```python
from build123d import *

# Parameters (mm, degrees)
F0_R     = 2.0193
F0_R_2   = 3.175
F1_DEPTH = 6.096
F2_R     = 3.175
F3_DEPTH = 25.401
F4_R     = 2.3876
F5_DEPTH = 34.926
F6_SIZE  = 2.54


with BuildPart() as f1:
    # F0 (on Front) → F1 (new body, symmetric)
    with BuildSketch(Plane.XZ):
        with BuildLine():
            Line((0, -63.5), (0, 0))
            Line((0, 0), (-10.16, 0))
            Line((-10.16, 0), (-10.16, -15.875))
            Line((-10.16, -15.875), (-12.7, -15.875))
            Line((-12.7, -15.875), (-12.7, -28.575))
            Line((-12.7, -28.575), (-25.4, -28.575))
            Line((-25.4, -28.575), (-25.4, -34.925))
            Line((-25.4, -34.925), (-15.875, -34.925))
            ThreePointArc((-15.875, -34.925), (-13.6299359697, -35.8549359697), (-12.7, -38.1))
            Line((-12.7, -38.1), (-12.7, -63.5))
            Line((-12.7, -63.5), (0, -63.5))
        make_face()
        with Locations((-6.35, -57.15)):
            Circle(F0_R, mode=Mode.SUBTRACT)
        with Locations((-6.35, -41.275)):
            Circle(F0_R_2, mode=Mode.SUBTRACT)
    extrude(amount=F1_DEPTH, both=True)

    # F2 (on face) → F3 (cut, through all)
    with BuildSketch(Plane.YZ):
        with Locations((0, -25.4)):
            Circle(F2_R)
        with Locations((0, -50.8)):
            Circle(F2_R)
    extrude(amount=-F3_DEPTH, mode=Mode.SUBTRACT)

    # F4 (on face) → F5 (cut, through all)
    with BuildSketch(Plane.XY.offset(-28.575)):
        with Locations((-19.05, 0)):
            Circle(F4_R)
    extrude(amount=-F5_DEPTH, mode=Mode.SUBTRACT)

    # F6
    f6_edges = [f1.edges().sort_by_distance(p)[0] for p in [
        (0, 0, 0),
    ]]
    chamfer(f6_edges, length=F6_SIZE)


solid = f1.part
```
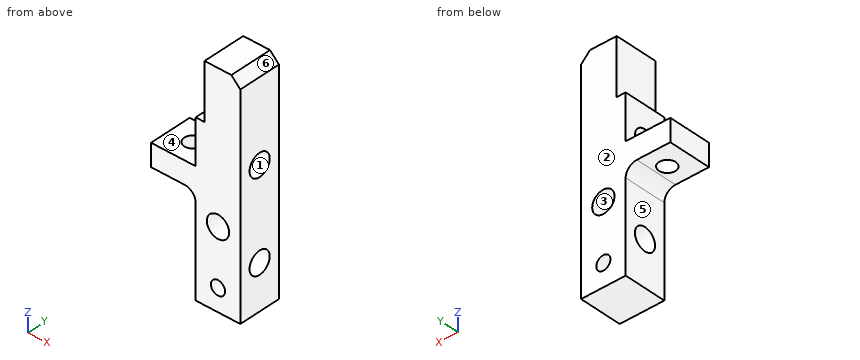
Input: part model. Units: mm. Frame: model coordinates. Face numbers are marked on the shaded views. A direction names the side the tool comes from. Give positions to 0.01 mm unless a question says otherwise; leave off trailing zeros. Write each loop counter-clockwise with the first axis right and the second up, starting at its lowest first coordinate (ties: lowest second). Pieces come first, ordered by that corner, then holes. Notation, with made-up numbers: (55.5, 19.25) - (112.5, 19.25) arc R23 ccw to (112.5, 51.25) - close; hole circle Ø8 at (75, 35.5). An arc over 180 degrees is marked (long way). Write item = value, one per line. Start each with the question number.
1) Material intervals for L1, parallel to Z at x = -6.35, y = -3.25; L2, parallel to Y at x = -9.25, z = -25.4 (3 decimals); L3, parallel to Z at x = -1.25, y = 2.75, sorted ascending. Write a range as [from, to].
2) Cut plane C-C (x = -6.25). Return loops of the section in (y, z) (3 decimals).
3) Draft query along Y for the marked faces 1, 2 and 3. Return one class per face: pulls with the +Y half, pulls with the -Y half, needs draft (parallel to the pull), parting line crosses it, or undercut.
4) Cut plane B-B (x = -19.05). Return loops of the section in (y, z) (3 decimals).
5) Reachability of the marked faces 4, 5 and 6 from +Z, -Z, +X, -X, +Y, -Y: full face, straight path, thin tool, end or side. Return the list, or none.
6) Cut plane D-D (y = 5). Return loops of the section in (x, z) (3 decimals).
7) Pin query (flat end, axial travel): pin 1 (1.3 mm diameter, centred on x = -11, y = 0, fed in from +Z) (3 decimals); pin 2 (6 mm diameter, centred on y = 0.5, z = -48, fed in from -X); pin 3 (5 mm diameter, centred on x = -18, y = 4.5, fed in from -Z). Return the tip coordinate at first contact, or that it passes through.
8) Cut plane A-A (z = -57.15). Return loops of the section in (x, y).
Answers follow:
q1.L1 = [-63.5, -59.17], [-55.13, -44.45], [-38.1, 0]
q1.L2 = [-6.096, -3.175], [3.175, 6.096]
q1.L3 = [-63.5, -52.39], [-49.21, -26.99], [-23.81, -1.29]
q2.outline = (-6.096, -63.5) - (6.096, -63.5) - (6.096, -59.167) - (-6.096, -59.167) - close; (-6.096, -55.133) - (6.096, -55.133) - (6.096, -44.448) - (-6.096, -44.448) - close; (-6.096, -38.102) - (6.096, -38.102) - (6.096, 0) - (-6.096, 0) - close; hole circle Ø6.35 at (0, -50.8); hole circle Ø6.35 at (0, -25.4)
q3.face_1 = undercut
q3.face_2 = pulls with the +Y half
q3.face_3 = needs draft
q4.outline = (-6.096, -34.925) - (-2.388, -34.925) - (-2.388, -28.575) - (-6.096, -28.575) - close; (2.388, -34.925) - (6.096, -34.925) - (6.096, -28.575) - (2.388, -28.575) - close
q5.face_4 = +Z, -X, +Y, -Y
q5.face_5 = -Z, -X, +Y, -Y
q5.face_6 = +Z, +X, +Y, -Y
q6.outline = (-25.4, -34.925) - (-15.875, -34.925) arc R3.175 cw to (-12.7, -38.1) - (-12.7, -63.5) - (0, -63.5) - (0, -2.54) - (-2.54, 0) - (-10.16, 0) - (-10.16, -15.875) - (-12.7, -15.875) - (-12.7, -28.575) - (-25.4, -28.575) - close; hole circle Ø6.35 at (-6.35, -41.275); hole circle Ø4.039 at (-6.35, -57.15)
q7.pin_1 = -15.875
q7.pin_2 = -12.7
q7.pin_3 = -34.95
q8.outline = (-12.7, -6.1) - (-8.37, -6.1) - (-8.37, 6.1) - (-12.7, 6.1) - close; (-4.33, -6.1) - (0, -6.1) - (0, 6.1) - (-4.33, 6.1) - close
